Verification items for the finished model (mm, model axes). Face numbers are marked on the shaded views. A direction names the side the tool comes from. Round coordinates to 2 decimals unless told otherwise and drop trailing zeros. Write each loop counter-clockwise with the first axis right and the second up, starting at its lowest first coordinate (ties: lowest second). Pieces come first, ordered by that corner, then holes. Notation, with made-up numbers: (47, 71.25) - (80, 71.25) arc R23 cw to (80, 100.25) - close; hole circle Ø6 at (38, 21). An arc over 180 degrees is marked (long way). Answer as a JSON object with one key per item and string values. Group by question number.
1) Mould release check, pull along Z, two halves, no side actions. Record for the marked faces 5, 6 and 7: +Z half, -Z half, draft (parallel to the pull), parting line (faces both ways), or undercut.
2) Set-up check for the marked faces 1, 2, 3 and 4: record each of +Z, -Z, +X, -X, +Y, -Y from which the full face is reachable in a straight line by a thin tool's end or side.
3) Section check B-B (z = 18.5). Enter the section's corners in (x, y).
4) Section check A-A (z = 42.5). Enter the section's corners in (x, y).
5) Thickness scan on line 1 (Y direction, x = -47.5, z = 38); line 2 (X direction, y = -8.5, z = 96); line 3 (X direction, y = 8.75, z = 14). Record the ranges inside material, lowest first.
6) Go/stop test with flat-tipped pins: pin 1 Ø6 at (y, z) = (4, 55.5) entering from -X; pin 2 Ø4 at (y, z) = (1.5, 89) entering from +X; pin 3 Ø1 at (y, z) = (8.5, 42.5) entering from -X. Record where each tip stops, or that it passes through.
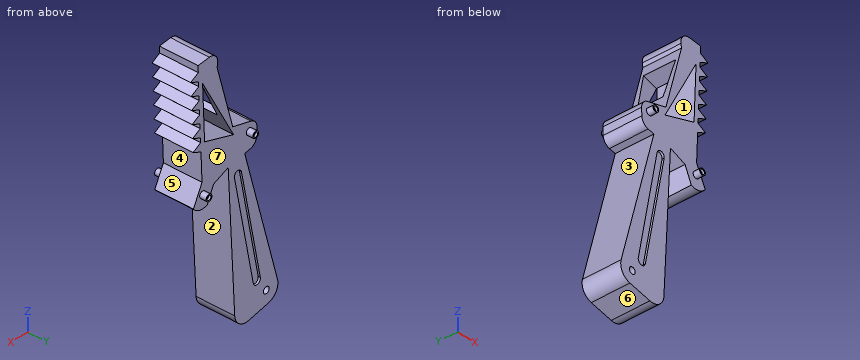
```python
from build123d import *

# Parameters (mm, degrees)
BOSS_EXTRUDE2_DEPTH = 9
FILLET2_R           = 6
FILLET3_R           = 4
BOSS_EXTRUDE3_DEPTH = 18
LPATTERN1_COUNT     = 6
LPATTERN1_PITCH     = 6
CUT_EXTRUDE1_DEPTH  = 26
CUT_EXTRUDE2_DEPTH  = 8
SKETCH6_R           = 1.5
CUT_EXTRUDE3_DEPTH  = 141.270424647
SKETCH7_R           = 1.5
BOSS_EXTRUDE4_DEPTH = 3
SKETCH8_R           = 1
CUT_EXTRUDE4_DEPTH  = 1
SKETCH9_R           = 1
CUT_EXTRUDE5_DEPTH  = 1
CUT_EXTRUDE6_DEPTH  = 1


with BuildPart() as part:
    # Sketch2 → Boss-Extrude2 (new, symmetric)
    with BuildSketch(Plane(origin=(0, 0, 0), x_dir=(1, 0, 0), z_dir=(0, 1, 0))):
        with BuildLine():
            ThreePointArc((-29.221908411, -61.269670629), (-25.308747509, -60.930081396), (-22.024034304, -63.083870674))
            Line((-22.024034304, -63.083870674), (-26.48393122, -72.034251644))
            Line((-26.48393122, -72.034251644), (-24.427510733, -121.991945093))
            Line((-24.427510733, -121.991945093), (-35.374328657, -123.072304919))
            Line((-35.374328657, -123.072304919), (-34.306141095, -116.154286754))
            Line((-34.306141095, -116.154286754), (-42.387240047, -87.26318363))
            Line((-42.387240047, -87.26318363), (-54.992342236, -84.083341057))
            Line((-54.992342236, -84.083341057), (-54.772056901, -74.085767632))
            Line((-54.772056901, -74.085767632), (-40.025552486, -71.339750966))
            Line((-40.025552486, -71.339750966), (-32.461637172, -68.287082299))
            Line((-32.461637172, -68.287082299), (-29.221908411, -61.269670629))
        make_face()
        Polygon((-40.025552486, -71.339750966), (-43.775331208, -0.438840115), (-67.242664489, -5.467186629), (-48.571202968, -72.931077154), align=None)
    extrude(amount=BOSS_EXTRUDE2_DEPTH, both=True)

    # Fillet2
    fillet2_edges = [part.edges().sort_by_distance(p)[0] for p in [
        (-67.242664489, 0, 5.467186629),
        (-43.775331208, 0, 0.438840115),
    ]]
    fillet(fillet2_edges, radius=FILLET2_R)

    # Fillet3
    fillet3_edges = [part.edges().sort_by_distance(p)[0] for p in [
        (-35.374328657, 0, 123.072304919),
        (-54.992342236, 0, 84.083341057),
        (-54.772056901, 0, 74.085767632),
    ]]
    fillet(fillet3_edges, radius=FILLET3_R)

    # Sketch3 → Boss-Extrude3 (add)
    with BuildSketch(Plane(origin=(0, 9, 0), x_dir=(1, 0, 0), z_dir=(0, 1, 0))):
        Polygon((-24.715653408, -114.991945093), (-24.633326929, -116.991945093), (-20.633326929, -116.827292136), align=None)
        Polygon((-24.633326929, -116.991945093), (-24.551000451, -118.991945093), (-20.633326929, -116.827292136), align=None)
    boss_extrude3 = extrude(amount=-BOSS_EXTRUDE3_DEPTH)

    # LPattern1: Boss-Extrude3 ×6
    with Locations(*[Vector(-0.04112840973087357, 0, -0.9991538689876598) * (i * LPATTERN1_PITCH) for i in range(1, LPATTERN1_COUNT)]):
        add(boss_extrude3)

    # Sketch4 → Cut-Extrude1 (cut)
    with BuildSketch(Plane(origin=(0, 9, 0), x_dir=(1, 0, 0), z_dir=(0, 1, 0))):
        Polygon((-26.777262548, -113.360971375), (-27.806343529, -88.360971375), (-42.806343529, -83.797470899), align=None)
    extrude(amount=-CUT_EXTRUDE1_DEPTH, mode=Mode.SUBTRACT)

    # Sketch5 → Cut-Extrude2 (cut)
    with BuildSketch(Plane(origin=(-61.948834437, 0, 17.327640931), x_dir=(0.2693699650610515, 0, 0.9630367708052524), z_dir=(-0.9630367708052524, 0, 0.2693699650610515))):
        Polygon((79.619805202, 6), (79.619805202, -6), (97.619805202, -7.510612388), (97.619805202, 7.510612388), align=None)
    extrude(amount=-CUT_EXTRUDE2_DEPTH, mode=Mode.SUBTRACT)

    # Sketch6 → Cut-Extrude3 (cut, through all)
    with BuildSketch(Plane(origin=(0, 9, 0), x_dir=(1, 0, 0), z_dir=(0, 1, 0))):
        with Locations(Location((-59.762437454, -10.000587386, 0), (0, 0, 270))):
            Circle(SKETCH6_R)
    extrude(amount=-CUT_EXTRUDE3_DEPTH, mode=Mode.SUBTRACT)

    # Sketch7 → Boss-Extrude4 (add)
    with BuildSketch(Plane(origin=(0, 9, 0), x_dir=(1, 0, 0), z_dir=(0, 1, 0))):
        with Locations(Location((-26.77516561, -66.748123847, 0), (0, 0, 270))):
            Circle(SKETCH7_R)
        with Locations(Location((-50.92309324, -80.984561831, 0), (0, 0, 270))):
            Circle(SKETCH7_R)
    boss_extrude4 = extrude(amount=BOSS_EXTRUDE4_DEPTH)

    # Sketch8 → Cut-Extrude4 (cut)
    with BuildSketch(Plane(origin=(0, 12, 0), x_dir=(1, 0, 0), z_dir=(0, 1, 0))):
        with Locations(Location((-50.92309324, -80.984561831, 0), (0, 0, 270))):
            Circle(SKETCH8_R)
    cut_extrude4 = extrude(amount=-CUT_EXTRUDE4_DEPTH, mode=Mode.SUBTRACT)

    # Sketch9 → Cut-Extrude5 (cut)
    with BuildSketch(Plane(origin=(0, 12, 0), x_dir=(1, 0, 0), z_dir=(0, 1, 0))):
        with Locations(Location((-26.77516561, -66.748123847, 0), (0, 0, 270))):
            Circle(SKETCH9_R)
    cut_extrude5 = extrude(amount=-CUT_EXTRUDE5_DEPTH, mode=Mode.SUBTRACT)

    # Sketch10 → Cut-Extrude6 (cut)
    with BuildSketch(Plane(origin=(0, 9, 0), x_dir=(1, 0, 0), z_dir=(0, 1, 0))):
        with BuildLine():
            Line((-53.032104668, -16.184151081), (-43.273460306, -65.40538361))
            ThreePointArc((-43.273460306, -65.40538361), (-44.729227788, -67.581140215), (-46.904984392, -66.125372733))
            Line((-46.904984392, -66.125372733), (-56.663628755, -16.904140204))
            ThreePointArc((-56.663628755, -16.904140204), (-55.207861273, -14.728383599), (-53.032104668, -16.184151081))
        make_face()
    cut_extrude6 = extrude(amount=-CUT_EXTRUDE6_DEPTH, mode=Mode.SUBTRACT)

    # Mirror1: Boss-Extrude4, Cut-Extrude4, Cut-Extrude5, Cut-Extrude6 across plane
    add(boss_extrude4.mirror(Plane.ZX))
    add(cut_extrude4.mirror(Plane.ZX), mode=Mode.SUBTRACT)
    add(cut_extrude5.mirror(Plane.ZX), mode=Mode.SUBTRACT)
    add(cut_extrude6.mirror(Plane.ZX), mode=Mode.SUBTRACT)


solid = part.part
```
Returned:
{
 "1": {"face 5": "undercut", "face 6": "-Z half", "face 7": "draft"},
 "2": {"face 1": "+Y, -Y", "face 2": "-Z, +Y, -Y", "face 3": "-X, +Y, -Y", "face 4": "+X, +Y, -Y"},
 "3": {"outline": "(-63.64, -9) - (-56.35, -9) - (-56.35, -8) - (-52.57, -8) - (-52.57, -9) - (-42.82, -9) - (-42.82, 9) - (-52.57, 9) - (-52.57, 8) - (-56.35, 8) - (-56.35, 9) - (-63.64, 9) - close"},
 "4": {"outline": "(-56.99, -9) - (-51.59, -9) - (-51.59, -8) - (-47.81, -8) - (-47.81, -9) - (-41.55, -9) - (-41.55, 9) - (-47.81, 9) - (-47.81, 8) - (-51.59, 8) - (-51.59, 9) - (-56.99, 9) - close"},
 "5": {"line 1": "-9 to 9", "line 2": "-39.94 to -36.19, -27.49 to -25.5", "line 3": "-64.88 to -43.06"},
 "6": {"pin 1": "x = -54.23", "pin 2": "x = -22.13", "pin 3": "x = -57.13"}
}
